Design review of the part shown in the three views and the two pictorial views. Dimensions are in mm from the part's minimum x, y and z. A direction names the side the tool comes from. Coordinates: 2 decimals unless noted, no trailing zeros. Write each loop counter-clockwise with the first axis right and the second up, starting at its lowest first coordinate (ties: lowest second). Pieces come first, ordered by that corner, then holes. Notation, with made-up numbers: (-38.5, 2) -> (9.5, 2) arc R15 cw to (9.5, 24) -> close; hole circle Ø11 at (34.25, -37). An arc over 180 degrees is marked (long way). Write item = value, one per line. Start each with the question number.
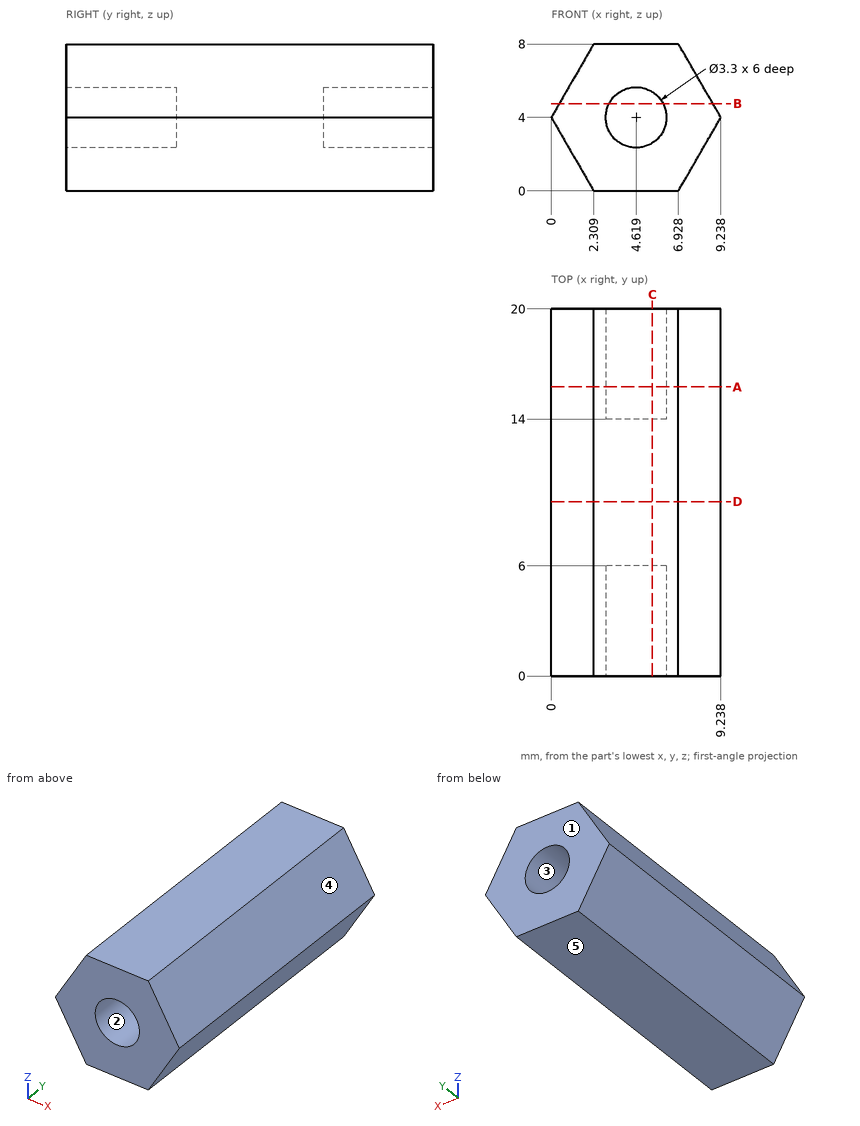
(1) Take a section at A-A, the plane y = 15.75. State the section outline as (x, z) points.
(2) Mouldability with a two-part tool opening along X and no side actions: class the marked faces 3, 4 and 5 as pulls with the +X half, pulls with the -X half, needs draft (parallel to the pull), parting line crosses it, or undercut.
(3) Take a section at D-D, the plane y = 9.5. State the section outline as (x, z) points.
(4) For the marked faces 1 and 2, list the 3-axis set-ups (+Z, -Z, +X, -X, +Y, -Y) from which the entire face can be reached by the end or side of a thin tool; tool diameter is ignored.
(5) Take a section at B-B, the plane z = 4.75. State the section outline as (x, y) points (1 decimal), then the cut area to 3 significant figures.
(6) For pin 1 Ø1 at (y, z) = (15, 7) entering from -X; pin 2 Ø2.5 at (x, z) = (4.62, 4) entering from +Y; pin 3 Ø4 at (y, z) = (17.5, 5) entering from -X, all flat-tipped, find the tip position at first contact; note any pin that passes through.
(7) Take a section at C-C, the plane x = 5.5. State the section outline as (y, z) points (1 decimal).
(8) For line 1 (X direction, y = 3.25, z = 2.5) (1 decimal); line 2 (Z direction, x = 5.5, y = 3) (1 decimal); line 3 (X direction, y = 4.5, z = 2.75) (1 decimal), list the stretches that pass through material, from the lowest coordinate up.
Report:
q1.outline = (0, 4) -> (2.31, 0) -> (6.93, 0) -> (9.24, 4) -> (6.93, 8) -> (2.31, 8) -> close; hole circle Ø3.3 at (4.62, 4)
q2.face_3 = undercut
q2.face_4 = pulls with the +X half
q2.face_5 = needs draft
q3.outline = (0, 4) -> (2.31, 0) -> (6.93, 0) -> (9.24, 4) -> (6.93, 8) -> (2.31, 8) -> close
q4.face_1 = +Z, -Z, +X, -X, +Y
q4.face_2 = -Y
q5.outline = (0.4, 0) -> (3.1, 0) -> (3.1, 6) -> (6.1, 6) -> (6.1, 0) -> (8.8, 0) -> (8.8, 20) -> (6.1, 20) -> (6.1, 14) -> (3.1, 14) -> (3.1, 20) -> (0.4, 20) -> close
q5.area = 132 mm2
q6.pin_1 = 1.44
q6.pin_2 = 14
q6.pin_3 = 0
q7.outline = (0, 0) -> (20, 0) -> (20, 2.6) -> (14, 2.6) -> (14, 5.4) -> (20, 5.4) -> (20, 8) -> (0, 8) -> (0, 5.4) -> (6, 5.4) -> (6, 2.6) -> (0, 2.6) -> close
q8.line_1 = 0.9 to 3.9, 5.3 to 8.4
q8.line_2 = 0 to 2.6, 5.4 to 8
q8.line_3 = 0.7 to 3.5, 5.7 to 8.5
